from build123d import *

# Parameters (mm, degrees)
SKETCH_1_W                = 90
SKETCH_1_H                = 70
SKETCH_1_W_2              = 86
SKETCH_1_H_2              = 66
EXTRUDE_1_DEPTH           = 22
SKETCH_2_W                = 90
SKETCH_2_H                = 70
EXTRUDE_2_DEPTH           = 2
CUT_EXTRUDE_1_DEPTH       = 1
CUT_EXTRUDE_1_DEPTH_BACK  = 91
SKETCH_4_R                = 1.5
CUT_EXTRUDE_2_DEPTH       = 1
CUT_EXTRUDE_2_DEPTH_BACK  = 91
CUT_EXTRUDE_3_DEPTH       = 21
CUT_EXTRUDE_3_DEPTH_BACK  = 3
SKETCH_7_R                = 1.9
SKETCH_7_R_2              = 1.6
CUT_EXTRUDE_4_DEPTH       = 1
CUT_EXTRUDE_4_DEPTH_BACK  = 71
SKETCH_9_R                = 1.1
CUT_EXTRUDE_5_DEPTH       = 1
CUT_EXTRUDE_5_DEPTH_BACK  = 71
SKETCH_10_R               = 3
SKETCH_10_R_2             = 1.6
EXTRUDE_3_DEPTH           = 2
SKETCH_11_R               = 3
SKETCH_11_R_2             = 1.6
EXTRUDE_4_DEPTH           = 2
SKETCH_12_R               = 1.6
CUT_EXTRUDE_6_DEPTH       = 1
CUT_EXTRUDE_6_DEPTH_BACK  = 23
SKETCH_16_W               = 11
SKETCH_16_H               = 27
CUT_EXTRUDE_9_DEPTH       = 1
CUT_EXTRUDE_9_DEPTH_BACK  = 91
SKETCH_17_W               = 45
SKETCH_17_H               = 27
EXTRUDE_6_DEPTH           = 2
FILLET_1_R                = 3
CUT_EXTRUDE_10_DEPTH      = 89
CUT_EXTRUDE_10_DEPTH_BACK = 3


with BuildPart() as part:
    # Эскиз1 → Бобышка-Вытянуть1 (new body)
    with BuildSketch(Plane.XY):
        Rectangle(SKETCH_1_W, SKETCH_1_H)
        Rectangle(SKETCH_1_W_2, SKETCH_1_H_2, mode=Mode.SUBTRACT)
    extrude(amount=EXTRUDE_1_DEPTH)

    # Эскиз2 → Бобышка-Вытянуть2 (add)
    with BuildSketch(Plane.XY.offset(22)):
        Rectangle(SKETCH_2_W, SKETCH_2_H)
    extrude(amount=-EXTRUDE_2_DEPTH)

    # Эскиз3 → Вырез-Вытянуть1 (cut, two sides)
    with BuildSketch(Plane.ZY.offset(45)) as cut_extrude_1_sk:
        with BuildLine():
            Line((17, 7.5), (17, -7.5))
            ThreePointArc((17, -7.5), (11, -13.5), (5, -7.5))
            Line((5, -7.5), (5, 7.5))
            ThreePointArc((5, 7.5), (11, 13.5), (17, 7.5))
        make_face()
    extrude(amount=CUT_EXTRUDE_1_DEPTH, mode=Mode.SUBTRACT)
    extrude(cut_extrude_1_sk.sketch, amount=-CUT_EXTRUDE_1_DEPTH_BACK, mode=Mode.SUBTRACT)

    # Эскиз4 → Вырез-Вытянуть2 (cut, two sides)
    with BuildSketch(Plane.ZY.offset(45)) as cut_extrude_2_sk:
        with Locations((11, 26)):
            Circle(SKETCH_4_R)
        with Locations((11, -26)):
            Circle(SKETCH_4_R)
    extrude(amount=CUT_EXTRUDE_2_DEPTH, mode=Mode.SUBTRACT)
    extrude(cut_extrude_2_sk.sketch, amount=-CUT_EXTRUDE_2_DEPTH_BACK, mode=Mode.SUBTRACT)

    # Эскиз5 → Вырез-Вытянуть3 (cut, two sides)
    with BuildSketch(Plane(origin=(0, 0, 20), x_dir=(-1, 0, 0), z_dir=(0, 0, -1))) as cut_extrude_3_sk:
        with BuildLine():
            Line((-10, 31), (-20, 31))
            ThreePointArc((-20, 31), (-21, 32), (-20, 33))
            Line((-20, 33), (-10, 33))
            ThreePointArc((-10, 33), (-9, 32), (-10, 31))
        make_face()
        with BuildLine():
            Line((10, 33), (20, 33))
            ThreePointArc((20, 33), (21, 32), (20, 31))
            Line((20, 31), (10, 31))
            ThreePointArc((10, 31), (9, 32), (10, 33))
        make_face()
        with BuildLine():
            Line((10, -31), (20, -31))
            ThreePointArc((20, -31), (21, -32), (20, -33))
            Line((20, -33), (10, -33))
            ThreePointArc((10, -33), (9, -32), (10, -31))
        make_face()
        with BuildLine():
            Line((-10, -33), (-20, -33))
            ThreePointArc((-20, -33), (-21, -32), (-20, -31))
            Line((-20, -31), (-10, -31))
            ThreePointArc((-10, -31), (-9, -32), (-10, -33))
        make_face()
    extrude(amount=CUT_EXTRUDE_3_DEPTH, mode=Mode.SUBTRACT)
    extrude(cut_extrude_3_sk.sketch, amount=-CUT_EXTRUDE_3_DEPTH_BACK, mode=Mode.SUBTRACT)

    # Эскиз7 → Вырез-Вытянуть4 (cut, two sides)
    with BuildSketch(Plane(origin=(0, 35, 0), x_dir=(1, 0, 0), z_dir=(0, 1, 0))) as cut_extrude_4_sk:
        with Locations((-37, -4)):
            Circle(SKETCH_7_R)
        with Locations((32.5, -4)):
            Circle(SKETCH_7_R_2)
    extrude(amount=CUT_EXTRUDE_4_DEPTH, mode=Mode.SUBTRACT)
    extrude(cut_extrude_4_sk.sketch, amount=-CUT_EXTRUDE_4_DEPTH_BACK, mode=Mode.SUBTRACT)

    # Эскиз9 → Вырез-Вытянуть5 (cut, two sides)
    with BuildSketch(Plane(origin=(0, 35, 0), x_dir=(1, 0, 0), z_dir=(0, 1, 0))) as cut_extrude_5_sk:
        with Locations((-32.5, -4)):
            Circle(SKETCH_9_R)
        with Locations((-41.5, -4)):
            Circle(SKETCH_9_R)
    extrude(amount=CUT_EXTRUDE_5_DEPTH, mode=Mode.SUBTRACT)
    extrude(cut_extrude_5_sk.sketch, amount=-CUT_EXTRUDE_5_DEPTH_BACK, mode=Mode.SUBTRACT)

    # Эскиз10 → Бобышка-Вытянуть3 (add)
    with BuildSketch(Plane(origin=(0, 35, 0), x_dir=(1, 0, 0), z_dir=(0, 1, 0))):
        with Locations((32.5, -4)):
            Circle(SKETCH_10_R)
        with Locations((32.5, -4)):
            Circle(SKETCH_10_R_2, mode=Mode.SUBTRACT)
    extrude(amount=EXTRUDE_3_DEPTH)

    # Эскиз11 → Бобышка-Вытянуть4 (add)
    with BuildSketch(Plane.XZ.offset(35)):
        with Locations((32.5, 4)):
            Circle(SKETCH_11_R)
        with Locations((32.5, 4)):
            Circle(SKETCH_11_R_2, mode=Mode.SUBTRACT)
    extrude(amount=EXTRUDE_4_DEPTH)

    # Эскиз12 → Вырез-Вытянуть6 (cut, two sides)
    with BuildSketch(Plane.XY.offset(22)) as cut_extrude_6_sk:
        with Locations((-32.5, 22.5)):
            Circle(SKETCH_12_R)
        with Locations((-32.5, -22.5)):
            Circle(SKETCH_12_R)
        with Locations((32.5, -22.5)):
            Circle(SKETCH_12_R)
        with Locations((32.5, 22.5)):
            Circle(SKETCH_12_R)
    extrude(amount=CUT_EXTRUDE_6_DEPTH, mode=Mode.SUBTRACT)
    extrude(cut_extrude_6_sk.sketch, amount=-CUT_EXTRUDE_6_DEPTH_BACK, mode=Mode.SUBTRACT)

    # Эскиз16 → Вырез-Вытянуть9 (cut, two sides)
    with BuildSketch(Plane(origin=(45, 0, 0), x_dir=(0, 0, -1), z_dir=(1, 0, 0))) as cut_extrude_9_sk:
        with Locations((-16.5, 0)):
            Rectangle(SKETCH_16_W, SKETCH_16_H)
    extrude(amount=CUT_EXTRUDE_9_DEPTH, mode=Mode.SUBTRACT)
    extrude(cut_extrude_9_sk.sketch, amount=-CUT_EXTRUDE_9_DEPTH_BACK, mode=Mode.SUBTRACT)

    # Эскиз17 → Бобышка-Вытянуть6 (add)
    with BuildSketch(Plane.XY.offset(22)):
        Rectangle(SKETCH_17_W, SKETCH_17_H)
    extrude(amount=-EXTRUDE_6_DEPTH)

    # Скругление1
    fillet_1_edges = [part.edges().sort_by_distance(p)[0] for p in [
        (-22.5, -13.5, 21),
        (-22.5, 13.5, 21),
        (22.5, 13.5, 21),
        (22.5, -13.5, 21),
    ]]
    fillet(fillet_1_edges, radius=FILLET_1_R)

    # Эскиз18 → Вырез-Вытянуть10 (cut, two sides)
    with BuildSketch(Plane.ZY.offset(-43)) as cut_extrude_10_sk:
        with BuildLine():
            Line((11, 13.5), (20, 13.5))
            Line((20, 13.5), (20, 33))
            Line((20, 33), (0, 33))
            Line((0, 33), (0, -33))
            Line((0, -33), (20, -33))
            Line((20, -33), (20, -13.5))
            Line((20, -13.5), (11, -13.5))
            ThreePointArc((11, -13.5), (6.757359313, -11.742640687), (5, -7.5))
            Line((5, -7.5), (5, 7.5))
            ThreePointArc((5, 7.5), (6.757359313, 11.742640687), (11, 13.5))
        make_face()
    extrude(amount=CUT_EXTRUDE_10_DEPTH, mode=Mode.SUBTRACT)
    extrude(cut_extrude_10_sk.sketch, amount=-CUT_EXTRUDE_10_DEPTH_BACK, mode=Mode.SUBTRACT)


solid = part.part
Can you work these out from the model? Positions are in its coordinate system, mm. A direction names the side the tool comes from. Give positions to 0.01 mm unless a question says otherwise; leave off trailing zeros. Loops run counter-clockwise (first coordinate to the right, second up) from the corner with the lowest first, then second, coordinate; pieces in that order, holes last. Notation, with made-up numbers: (46, 43) - (58, 43) arc R16 cw to (58, 50) - close; hole circle Ø6 at (62.25, 57.5). An arc over 180 degrees is marked (long way). One line per item, written item: value.
(1) On a 3-axis mill with a long thin cutter (end or side, diameter ignored), from which of +Z, -Z, +X, -X, +Y, -Y can I reach the whole of each face in a straight line? I mean faces 1 (the face through (-23.4, -12.64, 20.99)), 2 (the face through (29.5, -36, 4.1)), 3 (the face through (35, 13.5, 21)), 4 (the face through (-15, -31, 21)), 5 (the face through (34, 37, 5)). Say none if no direction works.
Verdict:
face 1: +Z, -Z, -X
face 2: -Y
face 3: +Z, -Z, +X
face 4: +Z, -Z
face 5: +Z, -Z, +X, -X, +Y
(2) If we section it at D-D, the plane x = 18: List the corners of the cut face in (y, z) for me, plus the area to 3 significant figures.
Verdict:
outline: (-35, 0) - (-33, 0) - (-33, 22) - (-35, 22) - close; (-31, 20) - (31, 20) - (31, 22) - (-31, 22) - close; (33, 0) - (35, 0) - (35, 22) - (33, 22) - close
area: 212 mm^2
(3) If we section it at C-C, the plane z = 18.5: List the corners of the cut face in (x, y) for me, plus the area to 3 significant figures.
Verdict:
outline: (-45, -35) - (45, -35) - (45, -33) - (-45, -33) - close; (-45, 33) - (45, 33) - (45, 35) - (-45, 35) - close
area: 360 mm^2
(4) If we mould it in two halves opening along X, with no side actions, what happens to faces 6 (the face through (-35, -13.5, 21)), 7 (the face through (-15, 31, 21)), 8 (the face through (-35.188, 34.014, 3.429)), 9 (the face through (29.5, 36, 3.9))? For each: released by +X, released by -X, zero draft, split by the parting line, or undercut.
Verdict:
face 6: zero draft
face 7: undercut
face 8: undercut
face 9: split by the parting line
(5) I need wall thicknesses on line 1 along Y through (x, z) = (-32.5, 20.85); line 2 along X through (y, z) = (-34.3, 4); line 3 along Y through (x, z) = (-0.5, 9). Which ranges of each line are inside material? Lowest first, please.
Verdict:
line 1: -35 to -24.1, -20.9 to -13.5, 13.5 to 20.9, 24.1 to 35
line 2: -45 to -42.6, -40.4 to -38.9, -35.1 to -33.6, -31.4 to 30.9, 34.1 to 45
line 3: -35 to -33, 33 to 35
(6) If we section it at A-A, the plane y = 32: List the corners of the cut face in (x, z) for me.
Verdict:
outline: (-45, 20) - (-21, 20) - (-21, 22) - (-45, 22) - close; (-9, 20) - (9, 20) - (9, 22) - (-9, 22) - close; (21, 20) - (45, 20) - (45, 22) - (21, 22) - close
(7) I'm going to push flat-ended pins straight in: pin 1 (0.6 mm diameter, centred on x = 13.5, z = 21, fed in from -Y); pin 2 (6 mm diameter, centred on x = -34.5, z = 11, fed in from +Y); pin 3 (20 mm diameter, centred on x = 14, y = -14.5, fed in from -Z). Where does each tip first touch, or does it pass through?
Verdict:
pin 1: y = -35
pin 2: y = 35
pin 3: z = 20
(8) If we section it at B-B, the plane x = -37: List the corners of the cut face in (y, z) for me.
Verdict:
outline: (-35, 0) - (-33, 0) - (-33, 2.1) - (-35, 2.1) - close; (-35, 5.9) - (-33, 5.9) - (-33, 20) - (-13.5, 20) - (-13.5, 22) - (-35, 22) - close; (13.5, 20) - (33, 20) - (33, 5.9) - (35, 5.9) - (35, 22) - (13.5, 22) - close; (33, 0) - (35, 0) - (35, 2.1) - (33, 2.1) - close
